Input: part model. Units: mm. Frame: model coordinates. A direction names the side the tool comes from. Give positions to 0.01 mm unless a question says otherwise; leave off trailing zeros. Loops run counter-clockwise (first coordinate to the right, second up) from the corner with the lowest first, then second, coordinate; pieces in that order, holes last. Notation, with made-up numbers: (75.5, 69) -> (89.5, 69) arc R22 ccw to (89.5, 91) -> close; hole circle Ø6 at (-6, 22.5). An arc over 180 degrees is marked (long way). Answer as a JSON object with one key per item and string values. Group by question number.
```python
from build123d import *

# Parameters (mm, degrees)
SKETCH1_R           = 25
BOSS_EXTRUDE1_DEPTH = 4.5
SKETCH2_R           = 12
BOSS_EXTRUDE2_DEPTH = 13
SKETCH3_R           = 7
CUT_EXTRUDE1_DEPTH  = 17.5
SKETCH4_R           = 2.5
CUT_EXTRUDE2_DEPTH  = 4.5
SKETCH5_R           = 2.5
CUT_EXTRUDE3_DEPTH  = 25
CIRPATTERN1_COUNT   = 2
CIRPATTERN1_ANGLE   = 90


with BuildPart() as part:
    # Sketch1 → Boss-Extrude1 (new body)
    with BuildSketch(Plane(origin=(0, 0, 0), x_dir=(1, 0, 0), z_dir=(0, 1, 0))):
        Circle(SKETCH1_R)
    extrude(amount=BOSS_EXTRUDE1_DEPTH)

    # Sketch2 → Boss-Extrude2 (add)
    with BuildSketch(Plane(origin=(0, 4.5, 0), x_dir=(1, 0, 0), z_dir=(0, 1, 0))):
        Circle(SKETCH2_R)
    extrude(amount=BOSS_EXTRUDE2_DEPTH)

    # Sketch3 → Cut-Extrude1 (cut)
    with BuildSketch(Plane(origin=(0, 17.5, 0), x_dir=(1, 0, 0), z_dir=(0, 1, 0))):
        Circle(SKETCH3_R)
    extrude(amount=-CUT_EXTRUDE1_DEPTH, mode=Mode.SUBTRACT)

    # Sketch4 → Cut-Extrude2 (cut)
    with BuildSketch(Plane(origin=(0, 4.5, 0), x_dir=(1, 0, 0), z_dir=(0, 1, 0))):
        with Locations((-18.5, 0)):
            Circle(SKETCH4_R)
        with Locations((0, 18.5)):
            Circle(SKETCH4_R)
        with Locations((18.5, 0)):
            Circle(SKETCH4_R)
        with Locations((0, -18.5)):
            Circle(SKETCH4_R)
    extrude(amount=-CUT_EXTRUDE2_DEPTH, mode=Mode.SUBTRACT)

    # Sketch5 → Cut-Extrude3 (cut)
    with BuildSketch(Plane(origin=(0, 0, 0), x_dir=(0.707106781, 0, 0.707106781), z_dir=(-0.707106781, 0, 0.707106781))):
        with Locations((0, 11)):
            Circle(SKETCH5_R)
    cut_extrude3 = extrude(amount=-CUT_EXTRUDE3_DEPTH, mode=Mode.SUBTRACT)

    # CirPattern1: Cut-Extrude3 ×2 about axis
    cirpattern1_axis = Axis((0, 17.5, 0), (0, 1, 0))
    for i in range(1, CIRPATTERN1_COUNT):
        add(cut_extrude3.rotate(cirpattern1_axis, i * CIRPATTERN1_ANGLE / (CIRPATTERN1_COUNT - 1)), mode=Mode.SUBTRACT)


solid = part.part
```
Q1. Section B-B on z = 0. Return the cut outline in (x, y).
Q2. Set-up query: faces 5 (the face through (-6, 4.5, 11)), 6 (the face through (5.2, 17.5, 5.2)). Return all of +Z, -Z, +X, -X, +Y, -Y with unobstructed straight access to the full face (end or side cutting, diameter ignored); none if empty.
Q3. Section C-C on y = 3.25. Return the cut outline in (x, z).
Q4. Ray query, probe 1 along X at (y, z) = (1.8, 0); probe 2 along Y at (x, z) = (-4, 16). Return the intervals inside material, ascending.
Q5. Section A-A on x = 0. Return the cut outline in (y, z), then the cut area to 3 significant figures.
Q6. Section D-D on y = 9.75. Return the cut outline in (x, z), then the cut area to 3 significant figures.
Q7. Pin query (flat end, axial travel): pin 1 Ø1 at (y, z) = (2.5, -18.5) entering from -X; pin 2 Ø10 at (y, z) = (13.5, 13.5) entering from +X; pin 3 Ø18 at (x, z) = (0, 0) entering from -Y; pin 4 Ø5 at (x, z) = (2, 2.5) entering from +Y. Return the tip coordinate at first contact, or that it passes through.
Q8. Pull-direction query (Z, two-part tool) for faces 1 (the face through (5.2, 0, 5.2)), 2 (the face through (-8.296, 11.11, -4.764)), 3 (the face through (11.085, 10.909, 4.596)), 4 (the face through (1.34, 2.28, 16.39)); classes: +Z half, -Z half, draft (parallel to the pull), parting line (faces both ways), or undercut.
Numbers:
{
 "1": {"outline": "(-25, 0) -> (-21, 0) -> (-21, 4.5) -> (-25, 4.5) -> close; (-16, 0) -> (-7, 0) -> (-7, 17.5) -> (-12, 17.5) -> (-12, 4.5) -> (-16, 4.5) -> close; (7, 0) -> (16, 0) -> (16, 4.5) -> (12, 4.5) -> (12, 17.5) -> (7, 17.5) -> close; (21, 0) -> (25, 0) -> (25, 4.5) -> (21, 4.5) -> close"},
 "2": {"face 5": "+Y", "face 6": "+Z, -Z, +X, -X, +Y"},
 "3": {"outline": "circle Ø50 at (0, 0); hole circle Ø5 at (-18.5, 0); hole circle Ø14 at (0, 0); hole circle Ø5 at (0, -18.5); hole circle Ø5 at (0, 18.5); hole circle Ø5 at (18.5, 0)"},
 "4": {"probe 1": "x = -25 to -21, -16 to -7, 7 to 16, 21 to 25", "probe 2": "y = 0 to 4.5"},
 "5": {"outline": "(0, -25) -> (4.5, -25) -> (4.5, -21) -> (0, -21) -> close; (0, -16) -> (4.5, -16) -> (4.5, -12) -> (17.5, -12) -> (17.5, -7) -> (0, -7) -> close; (0, 7) -> (17.5, 7) -> (17.5, 12) -> (4.5, 12) -> (4.5, 16) -> (0, 16) -> close; (0, 21) -> (4.5, 21) -> (4.5, 25) -> (0, 25) -> close", "area": "247 mm²"},
 "6": {"outline": "(-9.88, -6.82) -> (-6.24, -3.18) arc R7 cw (long way) to (6.24, -3.18) -> (9.88, -6.82) arc R12 ccw (long way) to start; (-6.82, -9.88) arc R12 ccw to (6.82, -9.88) -> (3.18, -6.24) arc R7 cw to (-3.18, -6.24) -> close", "area": "255 mm²"},
 "7": {"pin 1": "stops at x = -17.35", "pin 2": "stops at x = 8.47", "pin 3": "stops at y = 0", "pin 4": "passes through"},
 "8": {"face 1": "draft", "face 2": "undercut", "face 3": "parting line", "face 4": "undercut"}
}
